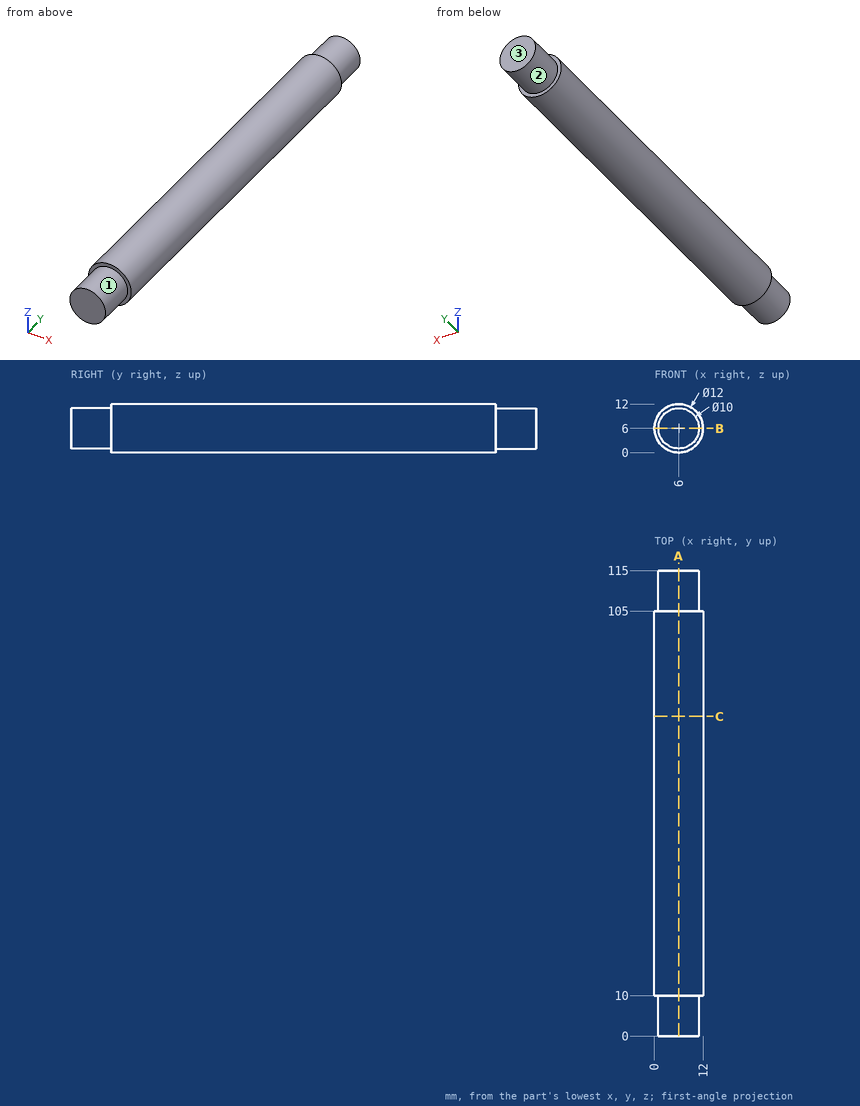
Could you check a few things on this drawing? It's one solid part, dimensions in mm from its lowest x, y, z. A direction names the side the tool comes from. Give positions to 0.01 mm unless a question says otherwise; leave off trailing zeros. Write each loop counter-clockwise with the first axis right and the second up, starting at its lowest first coordinate (ties: lowest second). Pieces come first, ordered by that corner, then holes. Notation, with made-up numbers: (-21, 6.25) -> (30, 6.25) arc R18 cw to (30, 16.25) -> close; hole circle Ø9 at (-1.75, 16.25). An arc over 180 degrees is marked (long way). Answer as CSV lines item,"result". Start each with the question number.
(1) If we section it at A-A, the plane x = 6: Write out the boundary of the cut face in (y, z), and give its area (3 significant figures).
(2) Please list where these lines run through material, in increasing order: line 1 (Y direction, x = 9.5, z = 10); line 2 (Z direction, x = 2.75, y = 92); line 3 (X direction, y = 18.5, z = 9).
(3) Which directions (+Z, -Z, +X, -X, +Y, -Y) give clear straight access to the entire face, cutting with the end or side of a thin tool? Please do the marked faces 1, 2 and 3.
(4) If we section it at B-B, the plane z = 6: Write out the boundary of the cut face in (x, y).
(5) If we section it at C-C, the plane y = 79: Write out the boundary of the cut face in (x, z).
(6) I'm going to push flat-ended pins straight in: pin 1 Ø5 at (x, z) = (7, 5.5) entering from -Y; pin 2 Ø5 at (y, z) = (18.5, 10) entering from -X; pin 3 Ø1 at (x, y) = (7, 26.5) entering from -Z; pin 4 Ø3 at (x, y) = (1.5, 71) entering from +Z. Where does each tip first touch, or does it pass through?
Answer list:
1,outline,"(0, 1) -> (10, 1) -> (10, 0) -> (105, 0) -> (105, 1) -> (115, 1) -> (115, 11) -> (105, 11) -> (105, 12) -> (10, 12) -> (10, 11) -> (0, 11) -> close"
1,area,"1,340 mm^2"
2,line 1,"10 to 105"
2,line 2,"0.96 to 11.04"
2,line 3,"0.8 to 11.2"
3,face 1,"-Y"
3,face 2,"+Y"
3,face 3,"+Z, -Z, +X, -X, +Y"
4,outline,"(0, 10) -> (1, 10) -> (1, 0) -> (11, 0) -> (11, 10) -> (12, 10) -> (12, 105) -> (11, 105) -> (11, 115) -> (1, 115) -> (1, 105) -> (0, 105) -> close"
5,outline,"circle Ø12 at (6, 6)"
6,pin 1,"y = 0"
6,pin 2,"x = 0.19"
6,pin 3,"z = 0.02"
6,pin 4,"z = 11.2"
